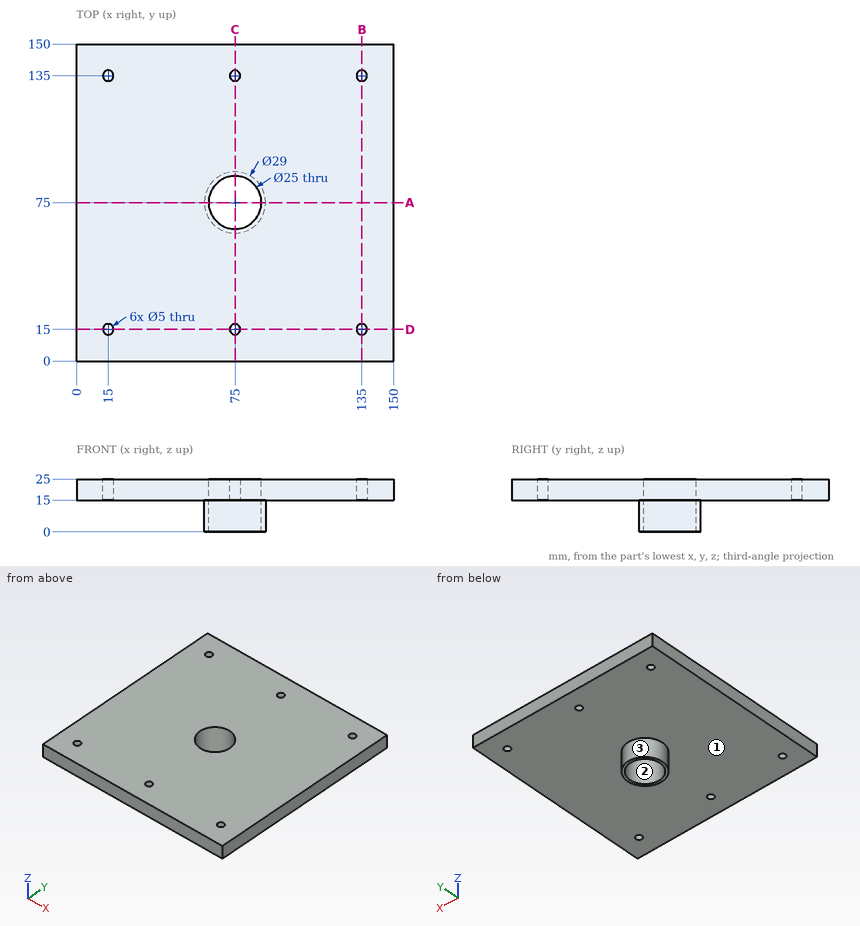
Could you check a few things on this drawing? It's one solid part, dimensions in mm from its lowest x, y, z. Coordinates: 2 decimals unless noted, no trailing zeros. Write each loop counter-clockwise with the first axis right and the second up, starting at its lowest first coordinate (ties: lowest second). Pieces come first, ordered by that corner, then holes. Notation, with made-up numbers: (61.25, -21) - (93.25, -21) arc R28 ccw to (93.25, 9) - close; hole circle Ø7 at (61, -15.5). An arc over 180 degrees is marked (long way). Return JSON: item names as keys, results as strings. Group by question number.
Item 1: If we section it at D-D (y = 15): Write out the boundary of the cut face in (x, z), then the cut area to 3 significant figures.
Item 2: Please list where these lines run through material, in increasing order: probe 1 along Y at (x, z) = (15, 21); probe 2 along Z at (x, y) = (107.5, 117); probe 3 along Y at (x, z) = (75, 13.75).
Item 3: I'm going to push flat-ended pins straight in: pin 1 Ø3 at (x, y) = (37, 132) entering from -Z; pin 2 Ø4 at (x, y) = (135, 15) entering from +Z. Where does each tip first touch, or does it pass through?
Item 4: If we section it at C-C (x = 75): Write out the boundary of the cut face in (y, z), then the cut area to 3 significant figures.
Item 5: If we section it at A-A (y = 75): Write out the boundary of the cut face in (x, z).
Item 6: If we section it at B-B (x = 135): Write out the boundary of the cut face in (y, z).
Item 7: We'd pull the mould along X, two halves only. Please class the marked faces 1, 2 and 3: pulls with the +X half, pulls with the -X half, needs draft (parallel to the pull), parting line crosses it, or undercut.
Return value:
{
 "1": {"outline": "(0, 15) - (12.5, 15) - (12.5, 25) - (0, 25) - close; (17.5, 15) - (72.5, 15) - (72.5, 25) - (17.5, 25) - close; (77.5, 15) - (132.5, 15) - (132.5, 25) - (77.5, 25) - close; (137.5, 15) - (150, 15) - (150, 25) - (137.5, 25) - close", "area": "1,350 mm^2"},
 "2": {"probe 1": "y = 0 to 12.5, 17.5 to 132.5, 137.5 to 150", "probe 2": "z = 15 to 25", "probe 3": "y = 60.5 to 62.5, 87.5 to 89.5"},
 "3": {"pin 1": "stops at z = 15", "pin 2": "passes through"},
 "4": {"outline": "(0, 15) - (12.5, 15) - (12.5, 25) - (0, 25) - close; (17.5, 15) - (60.5, 15) - (60.5, 0) - (62.5, 0) - (62.5, 25) - (17.5, 25) - close; (87.5, 0) - (89.5, 0) - (89.5, 15) - (132.5, 15) - (132.5, 25) - (87.5, 25) - close; (137.5, 15) - (150, 15) - (150, 25) - (137.5, 25) - close", "area": "1,210 mm^2"},
 "5": {"outline": "(0, 15) - (60.5, 15) - (60.5, 0) - (62.5, 0) - (62.5, 25) - (0, 25) - close; (87.5, 0) - (89.5, 0) - (89.5, 15) - (150, 15) - (150, 25) - (87.5, 25) - close"},
 "6": {"outline": "(0, 15) - (12.5, 15) - (12.5, 25) - (0, 25) - close; (17.5, 15) - (132.5, 15) - (132.5, 25) - (17.5, 25) - close; (137.5, 15) - (150, 15) - (150, 25) - (137.5, 25) - close"},
 "7": {"face 1": "needs draft", "face 2": "undercut", "face 3": "parting line crosses it"}
}
